Design review of the part built by this model. Coordinates are the model's own, in mm. A direction names the side the tool comes from. Give positions to 0.01 mm unless a question says otherwise; leave off trailing zeros. Write each loop counter-clockwise with the first axis right and the second up, starting at its lowest first coordinate (ties: lowest second). Pieces come first, ordered by that corner, then holes. Notation, with made-up numbers: M -16,49 L 3,49 A21 cw 3,77 Z; hole C 58,40 d4. An arc over 180 degrees is marked long. Write each question's results on one line, items separated by ' | '. Start each with the question number.
from build123d import *

# Parameters (mm, degrees)
BOSS_EXTRUDE1_DEPTH      = 1
BOSS_EXTRUDE1_DEPTH_BACK = 1
SKETCH1_R                = 1.6
BOSS_EXTRUDE4_START      = -2
BOSS_EXTRUDE4_DEPTH      = 2
FILLET1_R                = 3


with BuildPart() as part:
    # Sketch1 → Boss-Extrude1 (new, two sides: drawn at the far end of the back side and taken through both)
    with BuildSketch(Plane(origin=(0, 0, 0), x_dir=(1, 0, 0), z_dir=(0, 1, 0)).offset(-BOSS_EXTRUDE1_DEPTH_BACK)):
        with BuildLine():
            ThreePointArc((5, 11), (0, 16), (-5, 11))
            Line((-5, 11), (-5, -11))
            ThreePointArc((-5, -11), (0, -16), (5, -11))
            Line((5, -11), (5, 11))
        make_face()
        with Locations(Location((0, 11, 0), (0, 0, 270))):
            Circle(SKETCH1_R, mode=Mode.SUBTRACT)
        with Locations(Location((0, -11, 0), (0, 0, 270))):
            Circle(SKETCH1_R, mode=Mode.SUBTRACT)
    extrude(amount=BOSS_EXTRUDE1_DEPTH + BOSS_EXTRUDE1_DEPTH_BACK)

    # Sketch4 → Boss-Extrude4 (add)
    with BuildSketch(Plane(origin=(0, 1, 0), x_dir=(1, 0, 0), z_dir=(0, 1, 0)).offset(BOSS_EXTRUDE4_START)):
        with BuildLine():
            Line((2.958312472, 17.926759894), (-2.135268449, 15.521131346))
            ThreePointArc((-2.135268449, 15.521131346), (1.963819075, 15.59819689), (4.742555811, 12.58371853))
            Line((4.742555811, 12.58371853), (2.958312472, 17.926759894))
        make_face()
        with BuildLine():
            ThreePointArc((-5, 11), (-4.223525911, 13.676159352), (-2.135268449, 15.521131346))
            Line((-2.135268449, 15.521131346), (2.958312472, 17.926759894))
            Line((2.958312472, 17.926759894), (14.623518216, 23.436076894))
            Line((14.623518216, 23.436076894), (13.666416412, 25.462605676))
            Line((13.666416412, 25.462605676), (-5, 17.926759894))
            Line((-5, 17.926759894), (-5, 11))
        make_face()
    extrude(amount=BOSS_EXTRUDE4_DEPTH)

    # Fillet1
    # the kernel refuses this fillet: 3 mm, written as the material it adds along each edge
    with BuildSketch(Plane(origin=(2.958312472, -1, -17.926759894), x_dir=(0.9042262692177064, 0, -0.42705368989932413), z_dir=(0, 1, 0))) as fillet1_piece_1:
        with BuildLine():
            CenterArc((FILLET1_R * 0.887613530768, -FILLET1_R), FILLET1_R, 90, 83.185387179)
            Line((-FILLET1_R * 0.105321747078, -FILLET1_R * 0.881342787793), (0, 0))
            Line((0, 0), (FILLET1_R * 0.887613530768, 0))
        make_face()
    extrude(amount=2)
    # the kernel refuses this fillet: 3 mm, written as the material it takes off along each edge
    with BuildSketch(Plane(origin=(13.666416412, -7.931521676, -25.462605676), x_dir=(0.42705368989932463, 0, 0.904226269217706), z_dir=(0, 1, 0))) as fillet1_2_piece_1:
        with BuildLine():
            CenterArc((2.835616342, -2.940516757), FILLET1_R, 101.428639538, 75.275128979)
            Line((-0.159420459, -2.768021668), (0, 0))
            Line((0, 0), (2.241174417, 0))
        make_face()
    extrude(amount=15.863043352, mode=Mode.SUBTRACT)
    with BuildSketch(Plane(origin=(-5, -6.060290677, -17.926759894), x_dir=(0, 0, 1), z_dir=(0, 1, 0))) as fillet1_2_piece_2:
        with BuildLine():
            CenterArc((FILLET1_R * 0.674705423588, FILLET1_R), FILLET1_R, 201.984493206, 68.015506794)
            Line((-FILLET1_R * 0.252579782273, FILLET1_R * 0.625644357607), (0, 0))
            Line((0, 0), (FILLET1_R * 0.674705423588, 0))
        make_face()
    extrude(amount=12.120581354, mode=Mode.SUBTRACT)


solid = part.part
Q1. For faces 1 (the flat face through (4.28, -0.01, -13.97)), 2 (the cylindrical face through (0.07, -0.01, 9.4)), list the 3-axis set-ups (+Z, -Z, +X, -X, +Y, -Y) from which the entire face can be reached by the end or side of a thin tool; tool diameter is ignored.
Q2. For pin 1 Ø1.9 at (x, z) = (0, 11) entering from +Y; pin 2 Ø0.6 at (y, z) = (0.5, 3.5) entering from +X, all flat-tipped, find the tip position at first contact; note any pin that passes through.
Q3. We need section C-C on z = 5. Write out the cut boundary in (x, y), and give its area (3 significant figures).
Q4. We need section D-D on x = 10.5. Write out the cut boundary in (y, z).
Q5. We need section A-A on x = 1. Write out the cut boundary in (y, z), and give its area (3 significant figures).
Q6. Wall thickness on line 1 along X through (y, z) = (-0.5, -11); line 2 along X through (y, z) = (-0.05, -4.5); line 3 along Z through (x, y) = (10.5, 0.8): over which ranges is each line inside the solid? List them lowest first. Write a range as from..to.
Q7. The part is to be moulded in two halves that separate along Z. For faces 3 (the flat face through (5, 0, 0)), 4 (the flat face through (9.93, -0.01, -21.22)), 5 (the cylindrical face through (4.937, -0.014, -11.791)), 6 (the cylindrical face through (-4.473, -0.014, -17.601)), say which applies: pulls with the +Z half, pulls with the -Z half, needs draft (parallel to the pull), parting line crosses it, or undercut.
Q8. We need section B-B on y = 0.4. Write out the cut boundary in (x, z), and give its area (3 significant figures).
Answer sheet:
1) face 1: +X, +Y, -Y | face 2: +Y, -Y
2) pin 1: through | pin 2: x = 5
3) outline: M -5,-1 L 5,-1 L 5,1 L -5,1 Z | area: 20.0 mm^2
4) outline: M -1,-24.18 L 1,-24.18 L 1,-21.49 L -1,-21.49 Z
5) outline: M -1,-20.35 L 1,-20.35 L 1,-12.25 L -1,-12.25 Z; M -1,-9.75 L 1,-9.75 L 1,9.75 L -1,9.75 Z; M -1,12.25 L 1,12.25 L 1,15.9 L -1,15.9 Z | area: 62.5 mm^2
6) line 1: -5..-1.6, 1.6..5 | line 2: -5..5 | line 3: -24.18..-21.49
7) face 3: needs draft | face 4: pulls with the +Z half | face 5: undercut | face 6: pulls with the -Z half
8) outline: M -5,-15.9 A3 ccw -3.12,-18.68 L 11.1,-24.42 A3 ccw 14.62,-23.44 L 5.37,-19.06 A3 cw 3.8,-15.4 L 4.74,-12.58 A5 ccw 5,-11 L 5,11 A5 ccw -5,11 Z; hole C 0,-11 d3.2; hole C 0,11 d3.2 | area: 350 mm^2
